The listing builds one solid part. Answer for the finished solid, in the listing's coordinates (mm). A direction names the side the tool comes from. Give positions to 0.01 mm unless a question says otherwise; leave off trailing zeros. Loops run counter-clockwise (first coordinate to the right, second up) from the corner with the lowest first, then second, coordinate; pieces in that order, holes last. Notation, with made-up numbers: (-12.75, 76.5) - (40.25, 76.5) arc R14 ccw to (40.25, 95.5) - close; hole circle Ø2 at (35.5, 74). An arc over 180 degrees is marked (long way). Answer in a Markdown table with one row per item. Add a question column.
```python
from build123d import *

# Parameters (mm, degrees)
SKETCH2_R           = 10
BOSS_EXTRUDE1_DEPTH = 10
CUT_EXTRUDE1_START  = -11
CUT_EXTRUDE1_DEPTH  = 12
CIRPATTERN1_COUNT   = 14
FILLET1_R           = 0.25


with BuildPart() as part:
    # Sketch2 → Boss-Extrude1 (new body)
    with BuildSketch(Plane.XY):
        Circle(SKETCH2_R)
        with BuildLine():
            Line((2, 4.582575695), (2, 7))
            Line((2, 7), (-2, 7))
            Line((-2, 7), (-2, 4.582575695))
            ThreePointArc((-2, 4.582575695), (0, -5), (2, 4.582575695))
        make_face(mode=Mode.SUBTRACT)
    extrude(amount=BOSS_EXTRUDE1_DEPTH)

    # Sketch3 → Cut-Extrude1 (cut)
    with BuildSketch(Plane.XY.offset(10).offset(CUT_EXTRUDE1_START)):
        Polygon((-20.341084154, 62.326061337), (-1.266640021, 9.919456792), (-0.75, 8.5), (0.75, 8.5), (1.266640021, 9.919456792), (20.341084154, 62.326061337), (20.341084154, 173.86594871), (-20.341084154, 173.86594871), align=None)
    cut_extrude1 = extrude(amount=CUT_EXTRUDE1_DEPTH, mode=Mode.SUBTRACT)

    # CirPattern1: Cut-Extrude1 ×14 about axis
    cirpattern1_axis = Axis((0, 0, 0), (0, 0, 1))
    for i in range(1, CIRPATTERN1_COUNT):
        add(cut_extrude1.rotate(cirpattern1_axis, i * 360 / CIRPATTERN1_COUNT), mode=Mode.SUBTRACT)

    # Fillet1
    fillet1_edges = [part.edges().sort_by_distance(p)[0] for p in [
        (7.113184952, 4.713289704, 5),
        (6.17795025, 5.886036928, 5),
        (8.453777954, 1.160232004, 5),
        (8.119996553, 2.622623873, 5),
        (8.119996553, -2.622623873, 5),
        (8.453777954, -1.160232004, 5),
        (6.17795025, -5.886036928, 5),
        (7.113184952, -4.713289704, 5),
        (3.012285132, -7.983648182, 5),
        (4.363738433, -7.332822573, 5),
        (-0.75, -8.5, 5),
        (0.75, -8.5, 5),
        (-4.363738433, -7.332822573, 5),
        (-3.012285132, -7.983648182, 5),
        (-7.113184952, -4.713289704, 5),
        (-6.17795025, -5.886036928, 5),
        (-8.453777954, -1.160232004, 5),
        (-8.119996553, -2.622623873, 5),
        (-8.119996553, 2.622623873, 5),
        (-8.453777954, 1.160232004, 5),
        (-6.17795025, 5.886036928, 5),
        (-7.113184952, 4.713289704, 5),
        (-3.012285132, 7.983648182, 5),
        (-4.363738433, 7.332822573, 5),
        (4.363738433, 7.332822573, 5),
        (3.012285132, 7.983648182, 5),
        (0.75, 8.5, 5),
        (-0.75, 8.5, 5),
        (-1.266640021, 9.919456792, 5),
        (1.266640021, 9.919456792, 5),
        (5.445094229, 8.387547248, 5),
        (3.162687777, 9.486696265, 5),
        (-3.162687777, 9.486696265, 5),
        (-5.445094229, 8.387547248, 5),
        (-6.965606473, 7.174979196, 5),
        (-8.545080745, 5.194381104, 5),
        (-9.38890138, 3.442169501, 5),
        (-9.952609221, 0.972404078, 5),
        (-9.952609221, -0.972404078, 5),
        (-9.38890138, -3.442169501, 5),
        (-8.545080745, -5.194381104, 5),
        (-6.965606473, -7.174979196, 5),
        (-5.445094229, -8.387547248, 5),
        (-3.162687777, -9.486696265, 5),
        (-1.266640021, -9.919456792, 5),
        (1.266640021, -9.919456792, 5),
        (3.162687777, -9.486696265, 5),
        (5.445094229, -8.387547248, 5),
        (6.965606473, -7.174979196, 5),
        (8.545080745, -5.194381104, 5),
        (9.38890138, -3.442169501, 5),
        (9.952609221, -0.972404078, 5),
        (9.952609221, 0.972404078, 5),
        (9.38890138, 3.442169501, 5),
        (8.545080745, 5.194381104, 5),
        (6.965606473, 7.174979196, 5),
    ]]
    fillet(fillet1_edges, radius=FILLET1_R)


solid = part.part
```
(1) A cutting plane is placed at A-A on x = 0. Determine the outline of the cut face in (y, z), plus the area to 3 significant figures.
(2) A tool of negligible diameter and unlimited length cuts with its end or side. For faces 4 (the face through (-6.56, 6.51, 4.93)), 5 (the face through (-6.651, 5.293, 4.93)), 6 (the face through (-5, -2, 0)), 7 (the face through (4.889, 7.845, 4.93)), 8 (the face through (8.75, 3.03, 4.93)), from which of +Z, -Z, +X, -X, +Y, -Y can it reach the whole face along a straight path? Write none if from no direction.
(3) Given pin 1 Ø5 at (x, z) = (5, 3.5) entering from -Y; pin 2 Ø2.5 at (y, z) = (6.5, 4) entering from +X; pin 3 Ø1.5 at (x, z) = (-7, 8) entering from -Y; pin 4 Ø9 at (x, y) = (0, 0) entering from +Z, each flat-ended and moving along its own axis, determine where each tip first touches the part or whether it passes through.
(4) A cutting plane is placed at B-B on y = 0. Determine the outline of the cut face in (x, z), plus the area to 4 significant figures.
(5) Find the intervals of material crossed by line 1 along Y through (x, z) = (0, 2.5); line 2 along X through (y, z) = (8, 1.75); line 3 along Y through (x, z) = (5.5, 4), in increasing order. Write a range as [from, to].
(6) The mould has two halves that part along X. Classify faces 1 (the face through (-2.215, 9.752, 4.93)), 2 (the face through (-3.68, -7.66, 4.93)), 3 (the face through (6, 8, 5)): pulls with the +X half, pulls with the -X half, needs draft (parallel to the pull), parting line crosses it, or undercut.
Evaluation:
| question | item | result |
|---|---|---|
| 1 | outline | (-8.5, 0) - (-5, 0) - (-5, 10) - (-8.5, 10) - close; (7, 0) - (8.5, 0) - (8.5, 10) - (7, 10) - close |
| 1 | area | 50.0 mm² |
| 2 | face 4 | +Z, -Z, -X |
| 2 | face 5 | +Z, -Z |
| 2 | face 6 | -Z, +X, -X, +Y, -Y |
| 2 | face 7 | +Z, -Z, +Y |
| 2 | face 8 | +Z, -Z, +X |
| 3 | pin 1 | stops at y = -9.68 |
| 3 | pin 2 | stops at x = 6.9 |
| 3 | pin 3 | stops at y = -7.81 |
| 3 | pin 4 | passes through |
| 4 | outline | (-10, 0) - (-5, 0) - (-5, 10) - (-10, 10) - close; (5, 0) - (10, 0) - (10, 10) - (5, 10) - close |
| 4 | area | 100.0 mm² |
| 5 | line 1 | y = [-8.5, -5], [7, 8.5] |
| 5 | line 2 | x = [-6, -5.05], [-3.07, 3.07], [5.05, 6] |
| 5 | line 3 | y = [-8.32, 8.32] |
| 6 | face 1 | pulls with the -X half |
| 6 | face 2 | undercut |
| 6 | face 3 | pulls with the +X half |
